Design review of the part built by this model. Coordinates are the model's own, in mm. Face numbers are marked on the shaded views. Round coordinates to 2 decimals unless told otherwise and drop trailing zeros. Loops run counter-clockwise (first coordinate to the right, second up) from the corner with the lowest first, then second, coordinate; pieces in that order, holes last. Notation, with made-up numbers: (1.25, 29) - (28.25, 29) arc R20 ccw to (28.25, 33) - close; hole circle Ø4 at (-18.75, 2.5). An arc over 180 degrees is marked (long way). Answer as CSV lines item,"result". Start each with the question number.
(1) For P1, Ø1, axis at x = -53.5, y = 34, coming from the +Z side; P2, Ø4, axis at y = 15, z = -69.5, coming from the +X side; P3, Ø1, axis at x = -52, y = 33.5, coming from the -Z side; P4, Ø8, axis at x = -53.5, z = -2.5, coming from the -Y side, all flat-tipped, find the tip position at first contact; note any pin that passes through.
(2) Consider section B-B (z = -46). Give the boundary of the cut face in (x, y) (3 decimals).
(3) Consider section C-C (x = -32). Give the boundary of the cut face in (y, z) (3 decimals).
(4) Wall thickness on L1, parallel to X at y = 7.5, z = -49; L2, parallel to Z at x = -32, y = 33.5; L3, parallel to X at y = 19, z = -78: over which ranges is each line inside the solid? List them lowest first.
(5) Consider section D-D (y = 16). Give the boundary of the cut face in (x, z) (1 decimal), and give its area (3 significant figures).
(6) Consider section A-A (x = 11). Give the boundary of the cut face in (y, z) (3 decimals).
(7) Mouldability with a two-part tool opening along Z and no side actions: class the marked faces 1, 2 and 3 as released by +Z, released by -Z, zero draft, split by the parting line, or undercut.
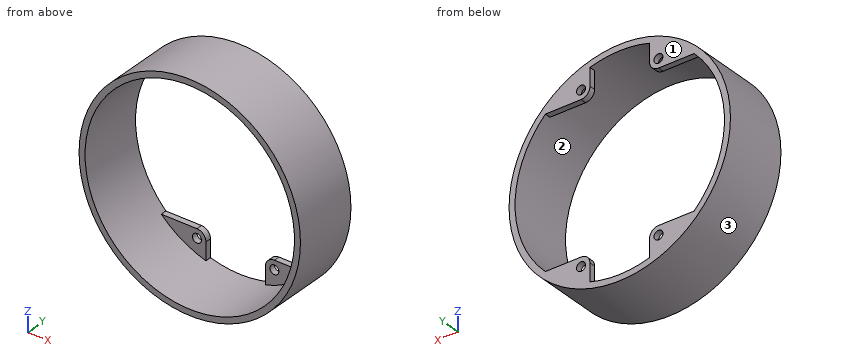
Autodesk Inventor part; units mm, degrees
ref_plane "YZ Plane" through (0, 0, 0) normal (1, 0, 0) x (0, 1, 0)
ref_plane "XZ Plane" through (0, 0, 0) normal (0, 1, 0) x (-1, 0, 0)
ref_plane "XY Plane" through (0, 0, 0) normal (0, 0, 1) x (1, 0, 0)
sketch "Sketch1" plane through (0, 0, 0) normal (0, 1, 0) x (-1, 0, 0)
  circle A0 centre (25.3149, -48.6245) radius 55.5625
  circle A1 centre (25.3149, -48.6245) radius 58.7375
  line L0 (0, -48.6245) -> (50.6298, -48.6245)
  line L1 (25.3149, -97.249) -> (25.3149, 0)
  circle A2 centre (45.8673, -4.7625) radius 2.3812
  circle A3 centre (4.7625, -4.7625) radius 2.3812
  circle A4 centre (45.8673, -92.4865) radius 2.3813
  circle A5 centre (4.7625, -92.4865) radius 2.3813
  arc A6 (45.8673, -87.724) -> (41.1048, -92.4865) centre (45.8673, -92.4865) ccw
  arc A7 (41.1048, -4.7625) -> (45.8673, -9.525) centre (45.8673, -4.7625) ccw
  arc A8 (4.7625, -9.525) -> (9.525, -4.7625) centre (4.7625, -4.7625) ccw
  line L2 (41.1048, -4.7625) -> (41.1048, 4.6472)
  line L3 (45.8673, -9.525) -> (64.7917, -9.525)
  line L4 (9.525, -4.7625) -> (9.525, 4.6472)
  line L5 (4.7625, -9.525) -> (-14.162, -9.525)
  line L6 (4.7625, -87.724) -> (-14.162, -87.724)
  line L7 (9.525, -92.4865) -> (9.525, -101.8962)
  line L8 (41.1048, -92.4865) -> (41.1048, -101.8961)
  line L9 (45.8673, -87.724) -> (64.7917, -87.724)
  arc A9 (9.525, -92.4865) -> (4.7625, -87.724) centre (4.7625, -92.4865) ccw
  point P0 (0, 0)
  dimension "d3" = 111.125
  dimension "d4" = 117.475
extrude "Extrusion1" add sketch "Sketch1" along normal blind 34.925 contours L3 A7 L2 A0 | A0 L8 A6 L9 | L4 A8 L5 A0 | A0 L6 A9 L7 | A1
extrude "Extrusion2" cut sketch "Sketch1" along normal blind 31.75 contours L3 A7 L2 A0 | A0 L8 A6 L9 | L4 A8 L5 A0 | A0 L6 A9 L7
properties part number "TxCeilingMount"
Determined:
1,P1,"stops at z = 3.18"
1,P2,"stops at x = 30.31"
1,P3,"stops at z = -101.2"
1,P4,"stops at y = 0"
2,outline,"(-83.994, 0) - (-80.815, 0) - (-80.815, 34.925) - (-83.994, 34.925) - close; (30.186, 0) - (33.364, 0) - (33.364, 34.925) - (30.186, 34.925) - close"
3,outline,"(0, -106.98) - (34.925, -106.98) - (34.925, -103.783) - (0, -103.783) - close; (0, 6.534) - (34.925, 6.534) - (34.925, 9.731) - (0, 9.731) - close"
4,L1,"x = -84.05 to -80.88, 30.25 to 33.42"
4,L2,"z = -106.98 to -103.78, 6.53 to 9.73"
4,L3,"x = -76.18 to -72.48, 21.85 to 25.55"
5,outline,"circle Ø117.5 at (-25.3, -48.6); hole circle Ø111.1 at (-25.3, -48.6)"
5,area,"1,140 mm^2"
6,outline,"(0, -94.791) - (34.925, -94.791) - (34.925, -87.724) - (31.75, -87.724) - (31.75, -90.677) - (0, -90.677) - close; (0, -6.572) - (31.75, -6.572) - (31.75, -9.525) - (34.925, -9.525) - (34.925, -2.458) - (0, -2.458) - close"
7,face 1,"zero draft"
7,face 2,"undercut"
7,face 3,"split by the parting line"
